Can you work these out from the drawing? Everything is in mm from the part's minimum corner. Give positions to 0.01 mm unless a question says otherwise; leave off trailing zeros. Write each loop counter-clockwise with the first axis right and the second up, starting at its lowest first coordinate (ties: lowest second). Pieces come first, ordered by that corner, then holes. Notation, with made-up numbers: M 2.5,-23 L 24.5,-23 A22 cw 24.5,-7 Z; hole C 21.5,81 d4. An arc over 180 degrees is marked long. One line per item, written item: value.
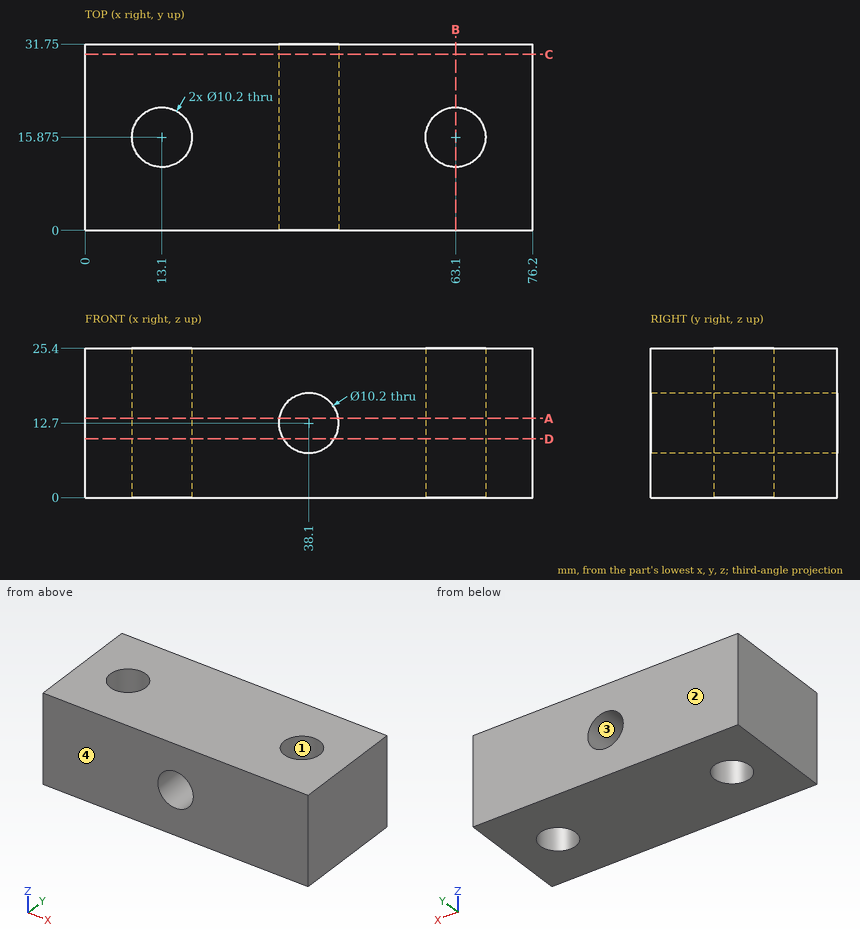
1) We'd pull the mould along Y, two halves only. Please class the marked faces 1, 2, 3 and 4: pulls with the +Y half, pulls with the -Y half, needs draft (parallel to the pull), parting line crosses it, or undercut.
Outcome:
face 1: undercut
face 2: pulls with the +Y half
face 3: needs draft
face 4: pulls with the -Y half
2) If we section it at A-A, the plane z = 13.5: Write out the boundary of the cut face in (x, y) (3 decimals), then the cut area to 3 significant figures.
Outcome:
outline: M 0,0 L 33.063,0 L 33.063,31.75 L 0,31.75 Z; M 43.137,0 L 76.2,0 L 76.2,31.75 L 43.137,31.75 Z; hole C 13.1,15.875 d10.2; hole C 63.1,15.875 d10.2
area: 1,940 mm^2
3) If we section it at B-B, the plane x = 63.1: Write out the boundary of the cut face in (y, z) (3 decimals).
Outcome:
outline: M 0,0 L 10.775,0 L 10.775,25.4 L 0,25.4 Z; M 20.975,0 L 31.75,0 L 31.75,25.4 L 20.975,25.4 Z
4) If we section it at D-D, the plane z = 10: Write out the boundary of the cut face in (x, y) (3 decimals), then the cut area to 3 significant figures.
Outcome:
outline: M 0,0 L 33.773,0 L 33.773,31.75 L 0,31.75 Z; M 42.427,0 L 76.2,0 L 76.2,31.75 L 42.427,31.75 Z; hole C 13.1,15.875 d10.2; hole C 63.1,15.875 d10.2
area: 1,980 mm^2
5) If we section it at C-C, the plane y = 30: Write out the boundary of the cut face in (x, z), then the cut area to 3 significant figures.
Outcome:
outline: M 0,0 L 76.2,0 L 76.2,25.4 L 0,25.4 Z; hole C 38.1,12.7 d10.2
area: 1,850 mm^2
6) Please list where these lines run through material, in increasing order: L1, parallel to X at y = 16, z = 12.75; L2, parallel to X at y = 15, z = 23; L3, parallel to Y at x = 63.1, z = 10 (3 decimals). Write a range as from..to.
Outcome:
L1: x = 0..8, 18.2..33, 43.2..58, 68.2..76.2
L2: x = 0..8.08, 18.12..58.08, 68.12..76.2
L3: y = 0..10.775, 20.975..31.75
